CAD build for the part. Positions are in the model's coordinates, mm. Face numbers are marked on the shaded views. A direction names the side the tool comes from. Coordinates: 2 decimals unless noted, no trailing zeros. Order: outer loops, then holes, each group sorted by start corner. A loop starts at its lowest first (then second) coordinate and runs counter-clockwise, first axis right, second up. Notation, with made-up numbers: M -40,56 L -31,56 A7 ccw -31,61 Z; hole C 6.25,24.25 d3. An arc over 180 degrees is marked long. One line per item, written item: value.
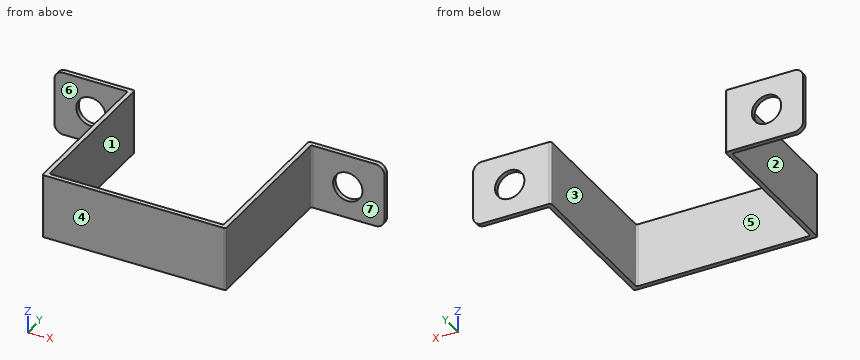
from build123d import *

# Parameters (mm, degrees)
F1_DEPTH = 7
F2_R     = 0.2
F3_R     = 1.6
F4_DEPTH = 0.501
F5_R     = 1


with BuildPart() as f1:
    # F0 (on Top) → F1 (new body)
    with BuildSketch(Plane.XY):
        Polygon((-10, 17), (-10, 0), (10, 0), (10, 17), (18, 17), (18, 17.5), (9.5, 17.5), (9.5, 0.5), (-9.5, 0.5), (-9.5, 17.5), (-18, 17.5), (-18, 17), align=None)
    extrude(amount=F1_DEPTH)

    # F2
    f2_edges = [f1.edges().sort_by_distance(p)[0] for p in [
        (10, 0, 3.5),
        (-10, 0, 3.5),
        (-9.5, 0.5, 3.5),
        (9.5, 0.5, 3.5),
        (-9.5, 17.5, 3.5),
        (-10, 17, 3.5),
        (10, 17, 3.5),
        (9.5, 17.5, 3.5),
    ]]
    fillet(f2_edges, radius=F2_R)

    # F3 (on face) → F4 (cut, through all)
    with BuildSketch(Plane.XZ.offset(-17)):
        with Locations((14, 3.5)):
            Circle(F3_R)
        with Locations((-14, 3.5)):
            Circle(F3_R)
    extrude(amount=-F4_DEPTH, mode=Mode.SUBTRACT)

    # F5
    f5_edges = [f1.edges().sort_by_distance(p)[0] for p in [
        (18, 17.25, 7),
        (18, 17.25, 0),
        (-18, 17.25, 7),
        (-18, 17.25, 0),
    ]]
    fillet(f5_edges, radius=F5_R)


solid = f1.part
Q1. Slice it at C-C (z = 3.5). List the corners of the cut face in (x, y).
Recorded:
outline: M -18,17 L -15.6,17 L -15.6,17.5 L -18,17.5 Z; M -12.4,17 L -10.2,17 A0.2 cw -10,16.8 L -10,0.2 A0.2 ccw -9.8,0 L 9.8,0 A0.2 ccw 10,0.2 L 10,16.8 A0.2 cw 10.2,17 L 12.4,17 L 12.4,17.5 L 9.7,17.5 A0.2 ccw 9.5,17.3 L 9.5,0.7 A0.2 cw 9.3,0.5 L -9.3,0.5 A0.2 cw -9.5,0.7 L -9.5,17.3 A0.2 ccw -9.7,17.5 L -12.4,17.5 Z; M 15.6,17 L 18,17 L 18,17.5 L 15.6,17.5 Z
Q2. Slice it at D-D (z = 0.5). List the corners of the cut face in (x, y), plus the area to 3 significant figures.
Recorded:
outline: M -17.87,17 L -10.2,17 A0.2 cw -10,16.8 L -10,0.2 A0.2 ccw -9.8,0 L 9.8,0 A0.2 ccw 10,0.2 L 10,16.8 A0.2 cw 10.2,17 L 17.87,17 L 17.87,17.5 L 9.7,17.5 A0.2 ccw 9.5,17.3 L 9.5,0.7 A0.2 cw 9.3,0.5 L -9.3,0.5 A0.2 cw -9.5,0.7 L -9.5,17.3 A0.2 ccw -9.7,17.5 L -17.87,17.5 Z
area: 34.9 mm^2
Q3. Slice it at B-B (x = 14). List the corners of the cut face in (y, z), plus the area to 3 significant figures.
Recorded:
outline: M 17,0 L 17.5,0 L 17.5,1.9 L 17,1.9 Z; M 17,5.1 L 17.5,5.1 L 17.5,7 L 17,7 Z
area: 1.90 mm^2
Q4. Which spindle directions (+Z, -Z, +X, -X, +Y, -Y) get a long thin tool onto all of the face, cutting with end or side? Do the marked faces 5, 6 and 7. Say none if no direction does.
Recorded:
face 5: +Z, -Z, +Y
face 6: +Z, -Z, -X, -Y
face 7: +Z, -Z, +X, -Y
Q5. Slice it at A-A (y = 12). List the corners of the cut face in (x, z), plus the area to 3 significant figures.
Recorded:
outline: M -10,0 L -9.5,0 L -9.5,7 L -10,7 Z; M 9.5,0 L 10,0 L 10,7 L 9.5,7 Z
area: 7.00 mm^2
Q6. Drill centre lines: line 1 along X through (y, z) = (16, 3); line 2 along Z through (x, y) = (-14, 17.4); line 3 along Y through (x, z) = (-8, 2). Where is each one in solid material? Low to high.
Recorded:
line 1: x = -10 to -9.5, 9.5 to 10
line 2: z = 0 to 1.9, 5.1 to 7
line 3: y = 0 to 0.5
Q7. Mould opens along X. For the marked faces 1, 2, 3 and 4 say: released by +X, released by -X, zero draft, split by the parting line, or undercut.
Recorded:
face 1: undercut
face 2: released by -X
face 3: undercut
face 4: zero draft
Q8. Pin check, flat tips, straight feed: pin 1 Ø3.5 at (y, z) = (7, 3.5) entering from +X; pin 2 Ø4 at (x, z) = (14, 3.5) entering from +Y; pin 3 Ø2 at (x, z) = (-4, 2.5) entering from +Y; pin 4 Ø3.5 at (y, z) = (5.5, 2.5) entering from -X. Stop position of each tip, or through.
Recorded:
pin 1: stops at x = 10
pin 2: stops at y = 17.5
pin 3: stops at y = 0.5
pin 4: stops at x = -10
